Work out the finished part from the listing and answer in its coordinate system (mm). A direction names the side the tool comes from. Give positions to 0.01 mm unless a question says otherwise; leave off trailing zeros. Loops run counter-clockwise (first coordinate to the right, second up) from the corner with the lowest first, then second, coordinate; pieces in that order, holes last. Notation, with made-up numbers: M 7,-28 L 11,-28 A13 cw 11,-18 Z; hole C 20.5,-20.5 d4. An arc over 180 degrees is marked long. Answer in a Markdown table with one row per item. Add a question column.
from build123d import *

# Parameters (mm, degrees)
SKETCH1_W           = 100
SKETCH1_H           = 40
SKETCH1_R           = 3.5
BOSS_EXTRUDE1_DEPTH = 6
SKETCH2_W           = 32
SKETCH2_H           = 40
BOSS_EXTRUDE2_DEPTH = 14
SKETCH3_W           = 20
SKETCH3_H           = 40
CUT_EXTRUDE1_DEPTH  = 14
FILLET2_R           = 5
FILLET3_R           = 5
BOSS_EXTRUDE3_DEPTH = 10
BOSS_EXTRUDE4_DEPTH = 10
SKETCH8_R           = 7.5
CUT_EXTRUDE2_DEPTH  = 29


with BuildPart() as part:
    # Sketch1 → Boss-Extrude1 (new body)
    with BuildSketch(Plane(origin=(0, 0, 0), x_dir=(1, 0, 0), z_dir=(0, 1, 0))):
        with Locations((-26.320522258, -4.639903709)):
            Rectangle(SKETCH1_W, SKETCH1_H)
        with Locations(Location((-66.320522258, 5.360096291, 0), (0, 0, 270))):
            Circle(SKETCH1_R, mode=Mode.SUBTRACT)
        with Locations(Location((-66.320522258, -14.639903709, 0), (0, 0, 270))):
            Circle(SKETCH1_R, mode=Mode.SUBTRACT)
        with Locations(Location((12.912927844, 5.360096291, 0), (0, 0, 270))):
            Circle(SKETCH1_R, mode=Mode.SUBTRACT)
        with Locations(Location((13.573914865, -14.639903709, 0), (0, 0, 270))):
            Circle(SKETCH1_R, mode=Mode.SUBTRACT)
    extrude(amount=BOSS_EXTRUDE1_DEPTH)

    # Sketch2 → Boss-Extrude2 (add)
    with BuildSketch(Plane(origin=(0, 6, 0), x_dir=(1, 0, 0), z_dir=(0, 1, 0))):
        with Locations((-26.320522258, -4.639903709)):
            Rectangle(SKETCH2_W, SKETCH2_H)
    extrude(amount=BOSS_EXTRUDE2_DEPTH)

    # Sketch3 → Cut-Extrude1 (cut)
    with BuildSketch(Plane.XZ):
        with Locations((-26.320522258, 4.639903709)):
            Rectangle(SKETCH3_W, SKETCH3_H)
    extrude(amount=-CUT_EXTRUDE1_DEPTH, mode=Mode.SUBTRACT)

    # Fillet2
    fillet2_edges = [part.edges().sort_by_distance(p)[0] for p in [
        (-36.320522258, 14, 4.639903709),
    ]]
    fillet(fillet2_edges, radius=FILLET2_R)

    # Fillet3
    fillet3_edges = [part.edges().sort_by_distance(p)[0] for p in [
        (-16.320522258, 14, 4.639903709),
    ]]
    fillet(fillet3_edges, radius=FILLET3_R)

    # Sketch6 → Boss-Extrude3 (add)
    with BuildSketch(Plane.XY.offset(9.639903709)):
        Polygon((-10.320522258, 6), (9.679477742, 6), (-10.320522258, 20), align=None)
        Polygon((-42.320522258, 6), (-62.320522258, 6), (-42.320522258, 20), align=None)
    extrude(amount=-BOSS_EXTRUDE3_DEPTH)

    # Sketch7 → Boss-Extrude4 (add)
    with BuildSketch(Plane(origin=(0, 20, 0), x_dir=(1, 0, 0), z_dir=(0, 1, 0))):
        with BuildLine():
            Line((-16.320522258, 2.860096291), (-16.320522258, -12.139903709))
            ThreePointArc((-16.320522258, -12.139903709), (-26.320522258, -22.139903709), (-36.320522258, -12.139903709))
            Line((-36.320522258, -12.139903709), (-36.320522258, 2.860096291))
            ThreePointArc((-36.320522258, 2.860096291), (-26.320522258, 12.860096291), (-16.320522258, 2.860096291))
        make_face()
    extrude(amount=BOSS_EXTRUDE4_DEPTH)

    # Sketch8 → Cut-Extrude2 (cut)
    with BuildSketch(Plane(origin=(-16.320522258, 0, 0), x_dir=(0, 0, -1), z_dir=(1, 0, 0))):
        with Locations((-4.639903709, 30)):
            Circle(SKETCH8_R)
    extrude(amount=-CUT_EXTRUDE2_DEPTH, mode=Mode.SUBTRACT)


solid = part.part
(1) Section C-C, the plane z = -6.5 is taken. Determine the outline of the cut face in (x, y).
(2) Section B-B, the plane x = 14.5 is taken. Determine the outline of the cut face in (y, z).
(3) Which of the six approach directions +Z, -Z, +X, -X, +Y, -Y give full straight-line access (tool end or side, diameter ignored) to faces 4 (the face through (-0.18, 12.9, 4.71)), 5 (the face through (-26, 14, 5)), 6 (the face through (-48, 10, -0.36)), 7 (the face through (-26.101, 24.93, 22.137)), 8 (the face through (-42.321, 13, 17))?
(4) The mould has two halves that part along X. Classify faces 1 (the face through (-48, 10, 9.64)), 2 (the face through (-42.321, 13, -8)), 3 (the face through (-34.89, 12.5, 4.92)): pulls with the +X half, pulls with the -X half, needs draft (parallel to the pull), parting line crosses it, or undercut.
(5) Consider line 1 along X through (y, z) = (4, 11); line 2 along Y through (x, z) = (-59.5, 17); line 3 along X through (y, z) = (9.25, -14). Determine where each line is inside the solid, lowest interval first. Write a range as from..to.
(6) Section A-A, the plane y = 27.25 is taken. Determine the outline of the cut face in (x, z).
(7) Section D-D, the plane y = 3.75 is taken. Determine the outline of the cut face in (x, z).
(8) Each of these flat-tipped pins is pushed along its axis until it touches: P1, Ø10, axis at x = -13.5, y = 22.5, coming from the -Z side; P2, Ø7, axis at x = -48, y = 15.5, coming from the -Z side; P3, Ø11, axis at y = 26, z = 4.5, coming from the -X side; P4, Ø5.5, axis at x = -66.32, z = 14.64, coming from the +Y side. Where does it stop, or does it pass through?
Numbers:
| question | item | result |
|---|---|---|
| 1 | outline | M -76.32,0 L -69.63,0 L -69.63,6 L -76.32,6 Z; M -63.01,0 L -36.32,0 L -36.32,9 A5 cw -31.32,14 L -21.32,14 A5 cw -16.32,9 L -16.32,0 L 9.6,0 L 9.6,6 L -10.32,6 L -10.32,20 L -17.01,20 L -17.01,30 L -35.63,30 L -35.63,20 L -42.32,20 L -42.32,6 L -63.01,6 Z; M 16.22,0 L 23.68,0 L 23.68,6 L 16.22,6 Z |
| 2 | outline | M 0,-15.36 L 6,-15.36 L 6,-8.48 L 0,-8.48 Z; M 0,-2.24 L 6,-2.24 L 6,11.26 L 0,11.26 Z; M 0,18.02 L 6,18.02 L 6,24.64 L 0,24.64 Z |
| 3 | face 4 | +Z, -Z, +X, +Y |
| 3 | face 5 | +Z, -Z, -Y |
| 3 | face 6 | -Z, -X, +Y |
| 3 | face 7 | +Z, +Y |
| 3 | face 8 | +Z, -X, +Y |
| 4 | face 1 | needs draft |
| 4 | face 2 | pulls with the -X half |
| 4 | face 3 | undercut |
| 5 | line 1 | x = -76.32..-36.32, -16.32..23.68 |
| 5 | line 2 | y = 0..6 |
| 5 | line 3 | x = -42.32..-36.31, -16.33..-10.32 |
| 6 | outline | M -36.32,-2.86 A10 ccw -16.32,-2.86 L -16.32,-2.34 L -36.32,-2.34 Z; M -36.32,11.62 L -16.32,11.62 L -16.32,12.14 A10 ccw -36.32,12.14 Z |
| 7 | outline | M -76.32,-15.36 L -36.32,-15.36 L -36.32,24.64 L -76.32,24.64 Z; M -16.32,-15.36 L 23.68,-15.36 L 23.68,24.64 L -16.32,24.64 Z; hole C -66.32,-5.36 d7; hole C -66.32,14.64 d7; hole C 12.91,-5.36 d7; hole C 13.57,14.64 d7 |
| 8 | P1 | stops at z = -15.36 |
| 8 | P2 | stops at z = -0.36 |
| 8 | P3 | stops at x = -36.32 |
| 8 | P4 | passes through |
